```python
from build123d import *

# Parameters (mm, degrees)
ESTRUSIONE_ESTRUSIONE1_DEPTH = 100
FORO_PER_VITE_M4_1_D         = 4.5
FORO_PER_VITE_M4_1_DEPTH     = 30
FORO_PER_VITE_M4_1_TIP       = 1.351936393


with BuildPart() as part:
    # Schizzo1 → Estrusione-Estrusione1 (new body)
    with BuildSketch(Plane.XY):
        with BuildLine():
            Line((-2.5, 0), (0, 0))
            Line((0, 0), (0, 10.5))
            Line((0, 10.5), (13, 10.5))
            Line((13, 10.5), (13, 13))
            Line((13, 13), (-10.5, 13))
            ThreePointArc((-10.5, 13), (-11.914213562, 13.585786438), (-12.5, 15))
            Line((-12.5, 15), (-12.5, 35))
            Line((-12.5, 35), (-14.5, 35))
            Line((-14.5, 35), (-14.5, 15))
            ThreePointArc((-14.5, 15), (-13.328427125, 12.171572875), (-10.5, 11))
            Line((-10.5, 11), (-2.5, 11))
            Line((-2.5, 11), (-2.5, 0))
        make_face()
    extrude(amount=ESTRUSIONE_ESTRUSIONE1_DEPTH)

    # Foro per Vite M4-1
    with Locations(Plane.ZY.offset(2.5)):
        with Locations((15, 4.5), (85, 4.5)):
            Hole(FORO_PER_VITE_M4_1_D / 2, depth=FORO_PER_VITE_M4_1_DEPTH)
            with Locations((0, 0, -(FORO_PER_VITE_M4_1_DEPTH + FORO_PER_VITE_M4_1_TIP / 2))):  # 118° drill point
                Cone(0, FORO_PER_VITE_M4_1_D / 2, FORO_PER_VITE_M4_1_TIP, mode=Mode.SUBTRACT)


solid = part.part
```
Geometry: final body of the model. Coordinates: model frame, mm. A direction names the side the tool comes from. Give positions to 0.01 mm unless a question says otherwise; leave off trailing zeros. Order: outer loops, then holes, each group sorted by start corner. A loop starts at its lowest first (then second) coordinate and runs counter-clockwise, first axis right, second up. Notation, with made-up numbers: M 42.5,28.5 L 89.5,28.5 A21 ccw 89.5,50.5 Z; hole C -35.5,66 d2. An arc over 180 degrees is marked long. Answer as CSV lines item,"result". Start each with the question number.
1) Cut plane D-D (z = 55.5). Output: boundary loops of the cut face in (x, y), then the cut area to 3 significant figures.
2) Set-up query: faces 1 (the flat face through (0, 5, 49)), 2 (the flat face through (-7, 11, 49)), 3 (the flat face through (1, 13, 49)). Return all of +Z, -Z, +X, -X, +Y, -Y with unobstructed straight access to the full face (end or side cutting, diameter ignored); none if empty.
3) Cut plane C-C (x = -1.5). Output: boundary loops of the cut face in (y, z).
4) Mould query, pull axis Y, two halves, no side actions, for faces 4 (the flat face through (6, 10.5, 49)), 5 (the cylindrical face through (-1.233, 5.176, 12.854)), 6 (the flat face through (-2.5, 6, 49)). Classes: +Y half, -Y half, draft (parallel to the pull), parting line (faces both ways), or undercut.
5) First-contact query: P1, Ø12, axis at x = -5.5, z = 57.5, coming from the +Y side; P2, Ø5, axis at y = 4.5, z = 85, coming from the +X side; P3, Ø3, axis at x = -8.5, z = 47, coming from the +Y side. Flat tips, straight axial feed; report the tip coordinate or a pass-through.
6) Cut plane B-B (y = 4.5). Output: boundary loops of the cut face in (x, z), then the cut area to 4 significant figures.
7) Line query: line 1 (Y direction, x = -1.7, z = 15); line 2 (X direction, y = 23, z = 28); line 3 (Y direction, x = 9.75, z = 86.5). Output: solid intervals per line, ascending. Write a range as from..to.
8) Cut plane A-A (z = 85). Output: boundary loops of the cut face in (x, y), then the cut area to 3 significant figures.
Findings below:
1,outline,"M -14.5,15 A4 ccw -10.5,11 L -2.5,11 L -2.5,0 L 0,0 L 0,10.5 L 13,10.5 L 13,13 L -10.5,13 A2 cw -12.5,15 L -12.5,35 L -14.5,35 Z"
1,area,"130 mm²"
2,face 1,"+Z, -Z, +X, -Y"
2,face 2,"+Z, -Z, -X, -Y"
2,face 3,"+Z, -Z, +X, +Y"
3,outline,"M 0,0 L 13,0 L 13,100 L 0,100 Z; hole C 4.5,15 d4.5; hole C 4.5,85 d4.5"
4,face 4,"-Y half"
4,face 5,"undercut"
4,face 6,"draft"
5,P1,"stops at y = 13.27"
5,P2,"stops at x = 0"
5,P3,"stops at y = 13"
6,outline,"M -2.5,0 L 0,0 L 0,12.75 L -2.5,12.75 Z; M -2.5,17.25 L 0,17.25 L 0,82.75 L -2.5,82.75 Z; M -2.5,87.25 L 0,87.25 L 0,100 L -2.5,100 Z"
6,area,"227.5 mm²"
7,line 1,"y = 0..2.25, 6.75..13"
7,line 2,"x = -14.5..-12.5"
7,line 3,"y = 10.5..13"
8,outline,"M -14.5,15 A4 ccw -10.5,11 L -2.5,11 L -2.5,6.75 L 0,6.75 L 0,10.5 L 13,10.5 L 13,13 L -10.5,13 A2 cw -12.5,15 L -12.5,35 L -14.5,35 Z; M -2.5,0 L 0,0 L 0,2.25 L -2.5,2.25 Z"
8,area,"119 mm²"
